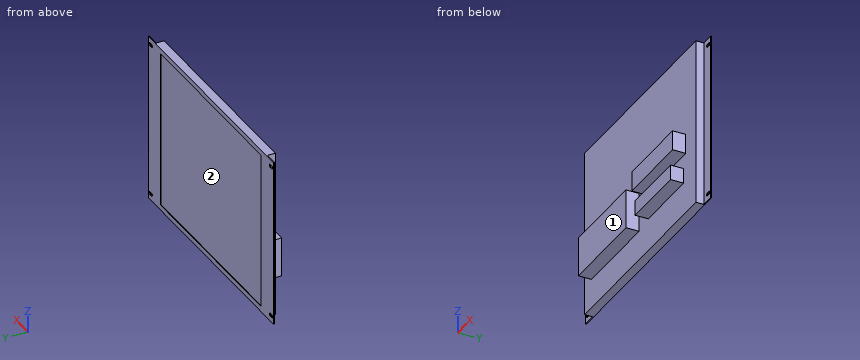
from build123d import *

# Parameters (mm, degrees)
SKETCH1_W           = 327
SKETCH1_H           = 256
BOSS_EXTRUDE1_DEPTH = 13.462
SKETCH2_W           = 20.25
SKETCH2_H           = 256
BOSS_EXTRUDE2_DEPTH = 1.5
SKETCH3_W           = 295.90708001
SKETCH3_H           = 240
CUT_EXTRUDE1_DEPTH  = 1
SKETCH4_W           = 140
SKETCH4_H           = 60
SKETCH4_W_2         = 120
SKETCH4_H_2         = 30
SKETCH4_W_3         = 104
SKETCH4_H_3         = 23
BOSS_EXTRUDE4_DEPTH = 20
CUT_EXTRUDE2_DEPTH  = 227.423867876


with BuildPart() as part:
    # Sketch1 → Boss-Extrude1 (new body)
    with BuildSketch(Plane(origin=(0, 0, 0), x_dir=(1, 0, 0), z_dir=(0, 1, 0))):
        Rectangle(SKETCH1_W, SKETCH1_H)
    extrude(amount=BOSS_EXTRUDE1_DEPTH)

    # Sketch2 → Boss-Extrude2 (add)
    with BuildSketch(Plane.XZ.offset(-13.462)):
        with Locations((173.625, 0)):
            Rectangle(SKETCH2_W, SKETCH2_H)
        with Locations((-173.625, 0)):
            Rectangle(SKETCH2_W, SKETCH2_H)
    extrude(amount=BOSS_EXTRUDE2_DEPTH)

    # Sketch3 → Cut-Extrude1 (cut)
    with BuildSketch(Plane(origin=(0, 13.462, 0), x_dir=(1, 0, 0), z_dir=(0, 1, 0))):
        Rectangle(SKETCH3_W, SKETCH3_H)
    extrude(amount=-CUT_EXTRUDE1_DEPTH, mode=Mode.SUBTRACT)

    # Sketch4 → Boss-Extrude4 (add)
    with BuildSketch(Plane.XZ):
        with Locations((-73.5, -53)):
            Rectangle(SKETCH4_W, SKETCH4_H)
        with Locations((73.5, -19)):
            Rectangle(SKETCH4_W_2, SKETCH4_H_2)
        with Locations((75.5, -66.5)):
            Rectangle(SKETCH4_W_3, SKETCH4_H_3)
    extrude(amount=BOSS_EXTRUDE4_DEPTH)

    # Sketch5 → Cut-Extrude2 (cut, through all)
    with BuildSketch(Plane(origin=(0, 13.462, 0), x_dir=(1, 0, 0), z_dir=(0, 1, 0))):
        with BuildLine():
            Line((174.375, 120.65), (179.125, 120.65))
            ThreePointArc((179.125, 120.65), (181.55, 118.225), (179.125, 115.8))
            Line((179.125, 115.8), (174.375, 115.8))
            ThreePointArc((174.375, 115.8), (171.95, 118.225), (174.375, 120.65))
        make_face()
        with BuildLine():
            Line((-179.125, 120.65), (-174.375, 120.65))
            ThreePointArc((-174.375, 120.65), (-171.95, 118.225), (-174.375, 115.8))
            Line((-174.375, 115.8), (-179.125, 115.8))
            ThreePointArc((-179.125, 115.8), (-181.55, 118.225), (-179.125, 120.65))
        make_face()
        with BuildLine():
            Line((-179.125, -115.5), (-174.375, -115.5))
            ThreePointArc((-174.375, -115.5), (-171.95, -117.925), (-174.375, -120.35))
            Line((-174.375, -120.35), (-179.125, -120.35))
            ThreePointArc((-179.125, -120.35), (-181.55, -117.925), (-179.125, -115.5))
        make_face()
        with BuildLine():
            Line((174.375, -115.5), (179.125, -115.5))
            ThreePointArc((179.125, -115.5), (181.55, -117.925), (179.125, -120.35))
            Line((179.125, -120.35), (174.375, -120.35))
            ThreePointArc((174.375, -120.35), (171.95, -117.925), (174.375, -115.5))
        make_face()
    extrude(amount=-CUT_EXTRUDE2_DEPTH, mode=Mode.SUBTRACT)


solid = part.part
Verification items for the finished model (mm, model axes). Face numbers are marked on the shaded views. Give positions to 0.01 mm unless a question says otherwise; leave off trailing zeros. Write each loop counter-clockwise with the first axis right and the second up, starting at its lowest first coordinate (ties: lowest second). Pieces come first, ordered by that corner, then holes. Notation, with made-up numbers: (7.5, 85) - (61.5, 85) arc R12 ccw to (61.5, 98) - close; hole circle Ø6 at (75, 78). An arc over 180 degrees is marked (long way). Answer as CSV lines item,"result". Start each with the question number.
1. Sectioned sample at B-B (x = -120.5). Record the boundary of the cut face in (y, z), then the cut area to 3 significant figures.
2. Depth check by flat-ended pin: pin 1 (6 mm diameter, centred on x = 99.5, y = -11, fed in from +Z); pin 2 (16 mm diameter, centred on x = 92.5, y = -11.5, fed in from -Z); pin 3 (8 mm diameter, centred on y = -8, z = -80, fed in from -X). Enter the tip coordinate at first touch or a pass-through.
3. Thickness scan on line 1 (X direction, y = -13.5, z = -56); line 2 (X direction, y = 7, z = -72); line 3 (Y direction, x = 69.5, z = 79.5). Record the ranges inside material, lowest first.
4. Sectioned sample at D-D (y = 8). Record the boundary of the cut face in (x, z), then the cut area to 3 significant figures.
5. Sectioned sample at C-C (z = 55). Record the boundary of the cut face in (x, y), then the cut area to 3 significant figures.
6. Draft check along X on the marked faces 1 and 2. Enter one of: pulls with the +X half, pulls with the -X half, needs draft (parallel to the pull), parting line crosses it, or undercut.
7. Sectioned sample at A-A (y = -11.5). Record the boundary of the cut face in (x, z), then the cut area to 3 significant figures.
Derived:
1,outline,"(-20, -83) - (0, -83) - (0, -128) - (13.46, -128) - (13.46, -120) - (12.46, -120) - (12.46, 120) - (13.46, 120) - (13.46, 128) - (0, 128) - (0, -23) - (-20, -23) - close"
1,area,"4,410 mm²"
2,pin 1,"z = -4"
2,pin 2,"z = -78"
2,pin 3,"x = -143.5"
3,line 1,"-143.5 to -3.5, 23.5 to 127.5"
3,line 2,"-163.5 to 163.5"
3,line 3,"0 to 12.46"
4,outline,"(-163.5, -128) - (163.5, -128) - (163.5, 128) - (-163.5, 128) - close"
4,area,"83,700 mm²"
5,outline,"(-183.75, 11.96) - (-163.5, 11.96) - (-163.5, 0) - (163.5, 0) - (163.5, 11.96) - (183.75, 11.96) - (183.75, 13.46) - (147.95, 13.46) - (147.95, 12.46) - (-147.95, 12.46) - (-147.95, 13.46) - (-183.75, 13.46) - close"
5,area,"4,170 mm²"
6,face 1,"needs draft"
6,face 2,"undercut"
7,outline,"(-143.5, -83) - (-3.5, -83) - (-3.5, -23) - (-143.5, -23) - close; (13.5, -34) - (133.5, -34) - (133.5, -4) - (13.5, -4) - close; (23.5, -78) - (127.5, -78) - (127.5, -55) - (23.5, -55) - close"
7,area,"14,400 mm²"
